from build123d import *

# Parameters (mm, degrees)
F1_DEPTH = 5
F2_R     = 2


with BuildPart() as f1:
    # F0 (on Top) → F1 (new body)
    with BuildSketch(Plane.XY):
        with BuildLine():
            ThreePointArc((-3, 5.6729591845), (0, 8.6729591845), (3, 5.6729591845))
            ThreePointArc((3, 5.6729591845), (2.7699992103, 4.5209590217), (2.1152637499, 3.5455994903))
            Line((2.1152637499, 3.5455994903), (-3.1437101653, -1.6834724502))
            ThreePointArc((-3.1437101653, -1.6834724502), (-1.9996201414, -2.073105577), (-0.8098901638, -2.2859401064))
            ThreePointArc((-0.8098901638, -2.2859401064), (0, -2.2494259195), (0.8098901638, -2.2859401064))
            ThreePointArc((0.8098901638, -2.2859401064), (3.4218298698, -1.5582979913), (5.640703333, 0))
            ThreePointArc((5.640703333, 0), (7.3866645607, 2.6009587503), (8, 5.6729591845))
            ThreePointArc((8, 5.6729591845), (0, 13.6729591845), (-8, 5.6729591845))
            Line((-8, 5.6729591845), (-3, 5.6729591845))
        make_face()
        with BuildLine():
            ThreePointArc((-0.8098901638, -2.2859401064), (-1.9996201414, -2.073105577), (-3.1437101653, -1.6834724502))
            Line((-3.1437101653, -1.6834724502), (-6.3457912496, -4.867346837))
            ThreePointArc((-6.3457912496, -4.867346837), (-3.8035324765, -3.0926409708), (-0.8098901638, -2.2859401064))
        make_face()
        with BuildLine():
            Line((2.8967557262, -2.7283458082), (5.640703333, 0))
            ThreePointArc((5.640703333, 0), (3.4218298698, -1.5582979913), (0.8098901638, -2.2859401064))
            ThreePointArc((0.8098901638, -2.2859401064), (1.8664770664, -2.4450938404), (2.8967557262, -2.7283458082))
        make_face()
        with BuildLine():
            ThreePointArc((0.8098901638, -2.2859401064), (0, -2.3270408155), (-0.8098901638, -2.2859401064))
            ThreePointArc((-0.8098901638, -2.2859401064), (-3.8035324765, -3.0926409708), (-6.3457912496, -4.867346837))
            ThreePointArc((-6.3457912496, -4.867346837), (-3.4560004885, -19.5594235503), (9, -11.2494259195))
            Line((9, -11.2494259195), (4, -11.2494259195))
            ThreePointArc((4, -11.2494259195), (-1.5360002171, -14.9427581999), (-2.8203516665, -8.4129463273))
            Line((-2.8203516665, -8.4129463273), (2.8967557262, -2.7283458082))
            ThreePointArc((2.8967557262, -2.7283458082), (1.8664770664, -2.4450938404), (0.8098901638, -2.2859401064))
        make_face()
    extrude(amount=F1_DEPTH)

    # F2
    f2_edges = [f1.edges().sort_by_distance(p)[0] for p in [
        (4, -11.249426, 2.5),
        (9, -11.249426, 2.5),
    ]]
    fillet(f2_edges, radius=F2_R)


solid = f1.part
For this review, take the finished solid that the model builds, in its own axes (mm). A direction names the side the tool comes from. Coordinates: 2 decimals unless noted, no trailing zeros. Loops run counter-clockwise (first coordinate to the right, second up) from the corner with the lowest first, then second, coordinate; pieces in that order, holes last. Notation, with made-up numbers: (78, 30) -> (125, 30) arc R16 ccw to (125, 47) -> close; hole circle Ø4 at (52.25, -4). An arc over 180 degrees is marked (long way). Write each question's results on one line, items separated by ' | '.
Q1. Add section C-C, the plane y = 7. State the section outline as (x, z) points.
Taken from the geometry:
outline: (-7.89, 0) -> (-2.69, 0) -> (-2.69, 5) -> (-7.89, 5) -> close; (2.69, 0) -> (7.89, 0) -> (7.89, 5) -> (2.69, 5) -> close
Q2. Add section D-D, the plane x = -3.5. State the section outline as (y, z) points, then the cut area to 3 significant figures.
Taken from the geometry:
outline: (-19.54, 0) -> (-13.19, 0) -> (-13.19, 5) -> (-19.54, 5) -> close; (-9.31, 0) -> (-2.04, 0) -> (-2.04, 5) -> (-9.31, 5) -> close; (5.67, 0) -> (12.87, 0) -> (12.87, 5) -> (5.67, 5) -> close | area: 104 mm²
Q3. Machinability: for faces 1 (the flat face through (6, -11.249, 2)), 2 (the cylindrical face through (4.516, -11.607, 2.535)), 3 (the flat face through (0, -3, 5)), 4 (the flat face through (-6, 5.673, 2)), which of the approach directions +Z, -Z, +X, -X, +Y, -Y give a long, thin tool a straight path to every point of the face, cutting with its end or side? Answer none if there is none.
Taken from the geometry:
face 1: +Z, -Z, +X | face 2: +Z, -Z | face 3: +Z, +X, -X, +Y, -Y | face 4: +Z, -Z, -X
Q4. To check wall thickness, follow line 1 along Y through (x, z) = (5.5, 4.2); line 2 along Y through (x, z) = (4.5, 4); line 3 along X through (y, z) = (6, 4.55). State the ranges of each line that lie inside material, in increasing order. Write a range as [from, to].
Taken from the geometry:
line 1: [-18.37, -11.26], [-0.14, 11.48] | line 2: [-19.04, -11.62], [-1.13, 12.29] | line 3: [-7.99, -2.98], [2.98, 7.99]
Q5. Add section A-A, the plane z = 3.7. State the section outline as (x, y) points, then the cut area to 3 significant figures.
Taken from the geometry:
outline: (-8, 5.67) -> (-3, 5.67) arc R3 cw (long way) to (2.12, 3.55) -> (-6.35, -4.87) arc R9 ccw (long way) to (8.62, -13.82) arc R2 ccw to (6.71, -11.25) -> (5.66, -11.25) arc R2 ccw to (3.77, -12.58) arc R4 cw (long way) to (-2.82, -8.41) -> (5.64, 0) arc R8 ccw (long way) to start; hole (-0.81, -2.29) arc R8 ccw to (0.81, -2.29) arc R9 ccw to start | area: 294 mm²
Q6. For pin 1 Ø6 at (x, y) = (-1, -7) entering from +Z; pin 2 Ø1.5 at (y, z) = (-13.5, 3.5) entering from -X; pin 3 Ø1 at (y, z) = (-2.5, 1.5) entering from +X, all flat-tipped, find the tip position at first contact; note any pin that passes through.
Taken from the geometry:
pin 1: z = 5 | pin 2: x = -8.87 | pin 3: x = 3.63
Q7. Add section B-B, the plane x = 5.25. State the section outline as (y, z) points.
Taken from the geometry:
outline: (-18.56, 0) -> (-11.29, 0) -> (-11.29, 5) -> (-18.56, 5) -> close; (-0.39, 0) -> (11.71, 0) -> (11.71, 5) -> (-0.39, 5) -> close
